Check sheet for the drawn part. Datum: minimum x, y, z corner. Units: mm. A direction names the side the tool comes from. Round coordinates to 2 decimals unless told otherwise and drop trailing zeros. Write each loop counter-clockwise with the first axis right and the second up, starting at its lowest first coordinate (ties: lowest second). Pieces come first, ordered by that corner, then holes. Notation, with made-up numbers: (65.5, 71.5) - (105.5, 71.5) arc R21 ccw to (105.5, 78.5) - close; hole circle Ø9 at (-34.75, 86.25). An arc over 180 degrees is marked (long way). Answer as a JSON object with one key per item and string values.
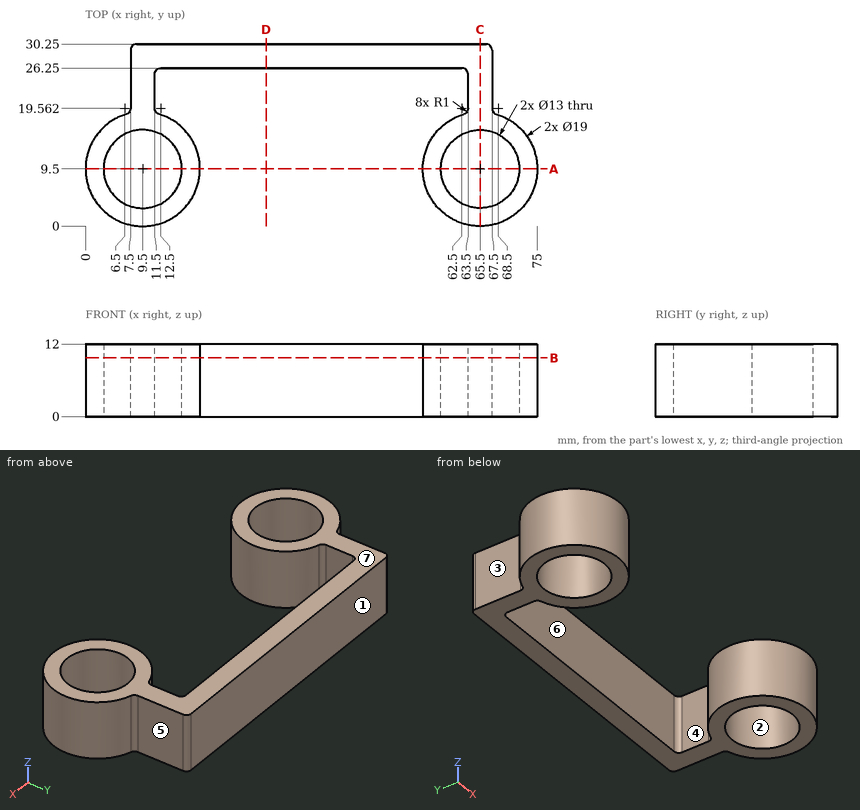
1. Go/stop test with flat-tipped pins: pin 1 (3 mm diameter, centred on x = 17, z = 10, fed in from -Y) (1 decimal); pin 2 (6.5 mm diameter, centred on y = 23, z = 6.5, fed in from -X); pin 3 (1.7 mm diameter, centred on y = 21.5, z = 3.5, fed in from +X). Record where each tip stops, or that it passes through.
Completed:
{"pin 1": "stops at y = 2.1", "pin 2": "stops at x = 7.5", "pin 3": "stops at x = 67.5"}
2. Cross-section at D-D (x = 30). Record the boundary of the cut face in (y, z), plus the area to 3 significant figures.
Completed:
{"outline": "(26.25, 0) - (30.25, 0) - (30.25, 12) - (26.25, 12) - close", "area": "48.0 mm^2"}
3. Cross-section at B-B (z = 9.75). Record the boundary of the cut face in (x, y).
Completed:
{"outline": "(6.79, 18.6) arc R9.5 ccw (long way) to (12.21, 18.6) arc R1 cw to (11.5, 19.56) - (11.5, 25.25) arc R1 cw to (12.5, 26.25) - (62.5, 26.25) arc R1 cw to (63.5, 25.25) - (63.5, 19.56) arc R1 cw to (62.79, 18.6) arc R9.5 ccw (long way) to (68.21, 18.6) arc R1 cw to (67.5, 19.56) - (67.5, 29.25) arc R1 ccw to (66.5, 30.25) - (8.5, 30.25) arc R1 ccw to (7.5, 29.25) - (7.5, 19.56) arc R1 cw to start; hole circle Ø13 at (9.5, 9.5); hole circle Ø13 at (65.5, 9.5)"}
4. Material ranges on probe 1 along Y at (x, z) = (65.5, 5); probe 2 along X at (y, z) = (6, 2.5); probe 3 along X at (y, z) = (7.5, 4.25) (1 decimal), recorded low to high. Write a range as from..to.
Completed:
{"probe 1": "y = 0..3, 16..30.25", "probe 2": "x = 0.67..4.02, 14.98..18.33, 56.67..60.02, 70.98..74.33", "probe 3": "x = 0.2..3.3, 15.7..18.8, 56.2..59.3, 71.7..74.8"}
5. Cross-section at A-A (y = 9.5). Record the boundary of the cut face in (x, z).
Completed:
{"outline": "(0, 0) - (3, 0) - (3, 12) - (0, 12) - close; (16, 0) - (19, 0) - (19, 12) - (16, 12) - close; (56, 0) - (59, 0) - (59, 12) - (56, 12) - close; (72, 0) - (75, 0) - (75, 12) - (72, 12) - close"}
6. Access from +Z, -Z, +X, -X, +Y, -Y to the whole of each face (thin tool, end or side, straight path). Record for the marked faces 5, 6 and 7.
Completed:
{"face 5": "+Z, -Z, +X, +Y", "face 6": "+Z, -Z", "face 7": "+Z, +X, -X, +Y, -Y"}
7. Cross-section at C-C (x = 65.5). Record the boundary of the cut face in (y, z).
Completed:
{"outline": "(0, 0) - (3, 0) - (3, 12) - (0, 12) - close; (16, 0) - (30.25, 0) - (30.25, 12) - (16, 12) - close"}
8. Mould release check, pull along Y, two halves, no side actions. Record for the marked faces 1, 2, 3 and 4: released by +Y, released by -Y, zero draft, split by the parting line, or undercut.
Completed:
{"face 1": "released by +Y", "face 2": "undercut", "face 3": "zero draft", "face 4": "undercut"}
